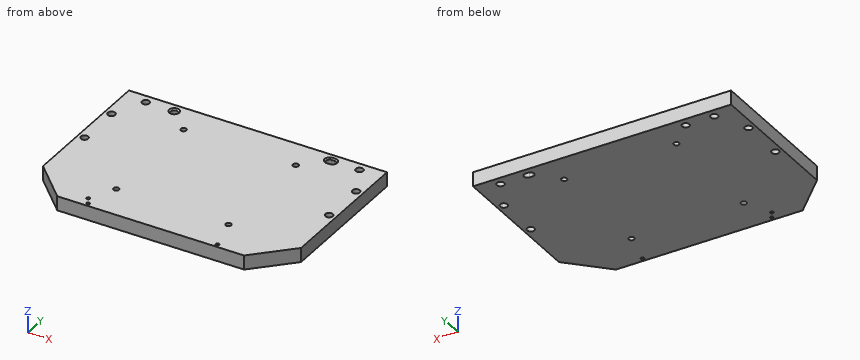
Autodesk Inventor part; units mm, degrees
ref_plane "YZ Plane" through (0, 0, 0) normal (1, 0, 0) x (0, 1, 0)
ref_plane "XZ Plane" through (0, 0, 0) normal (0, 1, 0) x (-1, 0, 0)
ref_plane "XY Plane" through (0, 0, 0) normal (0, 0, 1) x (1, 0, 0)
sketch "Sketch1" plane through (0, 0, 0) normal (0, 0, 1) x (1, 0, 0)
  line L0 (0, 111.252) -> (0, -111.887)
  line L1 (-161, 0) -> (161, 0)
  line L2 (115, -80.01) -> (-115, -80.01)
  line L3 (-115, -80.01) -> (-115, 79.375)
  line L4 (-115, 79.375) -> (115, 79.375)
  line L5 (115, 79.375) -> (115, -80.01)
  line L6 (50, -47.7648) -> (-50, -47.7648) construction
  line L7 (-50, -47.7648) -> (-50, 52.2352) construction
  line L8 (-50, 52.2352) -> (50, 52.2352) construction
  line L9 (50, 52.2352) -> (50, -47.7648) construction
  line L10 (50, -47.7648) -> (-50, 52.2352) construction
  line L11 (-50, -47.7648) -> (50, 52.2352) construction
  line L12 (109, 3.5) -> (-109, 3.5) construction
  line L13 (-109, 3.5) -> (-109, 43.5) construction
  line L14 (-109, 43.5) -> (109, 43.5) construction
  line L15 (109, 43.5) -> (109, 3.5) construction
  line L16 (109, 3.5) -> (-109, 43.5) construction
  line L17 (-109, 3.5) -> (109, 43.5) construction
  point P0 (0, 2.2352)
  point P1 (0, 23.5)
  point P2 (-57.62, -76.7648)
  point P3 (57.62, -76.7648)
  dimension "d0" = 230
  dimension "d1" = 159.385
  dimension "d4" = 100
  dimension "d5" = 100
  dimension "d28" = 35.875
  dimension "d29" = 40
  dimension "d30" = 6
  dimension "d38" = 29
  dimension "d39" = 79.375
  dimension "d40" = 115
  dimension "d48" = 2.2352
  dimension "d52" = 7.62
  dimension "d53" = 7.62
extrude "Extrusion1" add sketch "Sketch1" against normal blind 12.7
hole "Hole1" at (-50, 52.2352, 0) at (50, 52.2352, 0) at (50, -47.7648, 0) at (-50, -47.7648, 0) direction (0, 0, -1) diameter 4.9276 end through all
hole "Hole3" at (-109, 43.5, 0) at (-109, 3.5, 0) at (109, 3.5, 0) at (109, 43.5, 0) direction (0, 0, -1) diameter 6.604 end through all
chamfer "Chamfer1" distance 31.75 angle 45 2 edges at (-115, -80.01, -6.35) (115, -80.01, -6.35)
sketch "Sketch3" plane through (0, 0, -12.7) normal (0, 0, 1) x (1, 0, 0)
  line L0 (-95.25, 71.4375) -> (95.25, 71.4375) construction
  line L1 (0, 111.252) -> (0, -111.887) construction
  line L2 (-161, 0) -> (161, 0) construction
  line L3 (71.12, 71.4375) -> (68.58, 71.4375) construction
  line L4 (71.12, 74.6252) -> (68.58, 74.6252)
  line L5 (68.58, 68.2498) -> (71.12, 68.2498)
  arc A0 (71.12, 68.2498) -> (71.12, 74.6252) centre (71.12, 71.4375) ccw
  arc A1 (68.58, 74.6252) -> (68.58, 68.2498) centre (68.58, 71.4375) ccw
  line L6 (-115, 79.375) -> (115, 79.375)
  point P0 (0, 0)
  point P1 (-69.85, 71.4375)
  point P2 (69.85, 71.4375)
  dimension "d54" = 95.25
  dimension "d55" = 69.85
  dimension "d56" = 69.85
  dimension "d57" = 95.25
  dimension "d58" = 2.54
  dimension "d59" = 6.3754
  dimension "d69" = 7.9375
extrude "Extrusion3" cut sketch "Sketch3" along normal up to next
hole "Hole7" at (-69.85, 71.4375, -12.7) direction (0, 0, 1) diameter 6.3754 end through all
hole "Hole8" at (95.25, 71.4375, -12.7) at (-95.25, 71.4375, -12.7) direction (0, 0, 1) diameter 6.604 end through all
chamfer "Chamfer3" distance 1.27 angle 45 5 edges at (-69.85, 68.2498, 0) (65.3923, 71.4375, 0) (69.85, 74.6252, 0) (74.3077, 71.4375, 0) (69.85, 68.2498, 0)
sketch "Sketch4" plane through (0, 0, -12.7) normal (0, 0, -1) x (-1, 0, 0)
  line L0 (0, -111.887) -> (0, 111.252)
  line L1 (-161, 0) -> (161, 0)
  line L2 (60, -77.854) -> (-60, -77.854) construction
  line L3 (-60, -77.854) -> (-60, 77.854) construction
  line L4 (-60, 77.854) -> (60, 77.854) construction
  line L5 (60, 77.854) -> (60, -77.854) construction
  line L6 (60, -77.854) -> (-60, 77.854) construction
  line L7 (-60, -77.854) -> (60, 77.854) construction
  circle A0 centre (61.5, -70.4148) radius 1.5 construction
  point P0 (0, 0)
  point P1 (-57.62, -76.7648)
  point P2 (57.62, -76.7648)
  dimension "d106" = 120
  dimension "d107" = 3
  dimension "d108" = 6.35
hole "Hole9" at (57.62, -76.7648, -12.7) at (-57.62, -76.7648, -12.7) at (-61.5, -70.4148, -12.7) direction (0, 0, 1) diameter 2.9972 end through all counterbore diameter 3.0226 counterbore depth 1.905
equation "\"d40\" = 0.5 * d0"
equation "\"d57\" = d54"
properties part number "J008086" material "ALUMINUM, 6061-T651"
The model under review builds one solid part; all positions refer to its coordinate system, in mm. Round coordinates to 2 decimals unless told otherwise and drop trailing zeros. Loops run counter-clockwise (first coordinate to the right, second up) from the corner with the lowest first, then second, coordinate; pieces in that order, holes last. Notation, with made-up numbers: (25, 48.25) -> (51, 48.25) arc R14 ccw to (51, 70.25) -> close; hole circle Ø8 at (82.25, 36.25). An arc over 180 degrees is marked (long way). Answer as a JSON object with one key per item and string values. Group by question number.
1) For line 1 (Y direction, x = -50, z = -3) (3 decimals); line 2 (X direction, y = 71, z = -9.5); line 3 (Y direction, x = 109, z = -4.5) (3 decimals), list the stretches that pass through material, from the lowest coordinate up. Write a range as [from, to].
2) We need section C-C on y = 43.5. Write out the cut boundary in (x, z).
3) For pin 1 Ø4 at (x, y) = (-109, 3.5) entering from +Z; pin 2 Ø2 at (x, z) = (-91.5, -8) entering from -Y, all flat-tipped, find the tip position at first contact; note any pin that passes through.
4) We need section D-D on x = -95.25. Write out the cut boundary in (y, z) (1 decimal).
5) We need section B-B on z = -6. Give the number of separate pieces and of enclosed holes in the cut face, then the cut area to 3 significant figures.
6) We need section A-A on x = -50. Write out the cut boundary in (y, z) (3 decimals).
Result set:
{
 "1": {"line 1": "[-80.01, -50.229], [-45.301, 49.771], [54.699, 79.375]", "line 2": "[-115, -98.52], [-91.98, -73.01], [-66.69, 65.42], [74.28, 91.98], [98.52, 115]", "line 3": "[-54.26, 0.198], [6.802, 40.198], [46.802, 79.375]"},
 "2": {"outline": "(-115, -12.7) -> (-112.3, -12.7) -> (-112.3, 0) -> (-115, 0) -> close; (-105.7, -12.7) -> (105.7, -12.7) -> (105.7, 0) -> (-105.7, 0) -> close; (112.3, -12.7) -> (115, -12.7) -> (115, 0) -> (112.3, 0) -> close"},
 "3": {"pin 1": "through", "pin 2": "y = -72.76"},
 "4": {"outline": "(-68, -12.7) -> (68.1, -12.7) -> (68.1, 0) -> (-68, 0) -> close; (74.7, -12.7) -> (79.4, -12.7) -> (79.4, 0) -> (74.7, 0) -> close"},
 "5": {"separate pieces": "1", "enclosed holes": "15", "area": "35,300 mm²"},
 "6": {"outline": "(-80.01, -12.7) -> (-50.229, -12.7) -> (-50.229, 0) -> (-80.01, 0) -> close; (-45.301, -12.7) -> (49.771, -12.7) -> (49.771, 0) -> (-45.301, 0) -> close; (54.699, -12.7) -> (79.375, -12.7) -> (79.375, 0) -> (54.699, 0) -> close"}
}
